from build123d import *

# Parameters (mm, degrees)
F1_DEPTH = 3.175
F2_R     = 38.608
F2_R_2   = 36.322
F2_R_3   = 11.1633
F3_DEPTH = 1.524
F4_R     = 0.5334
F5_DEPTH = 3.176


with BuildPart() as f1:
    # F0 (on Top) → F1 (new body)
    with BuildSketch(Plane.XY):
        Polygon((18.411793, 44.45), (-18.411793, 44.45), (-44.45, 18.411793), (-44.45, 0), (44.45, 0), (44.45, 18.411793), align=None)
        Polygon((44.45, 0), (-44.45, 0), (-44.45, -18.411793), (-18.411793, -44.45), (18.411793, -44.45), (44.45, -18.411793), align=None)
    extrude(amount=F1_DEPTH)

    # F2 (on face) → F3 (cut)
    with BuildSketch(Plane.XY.offset(3.175)):
        Circle(F2_R)
        Circle(F2_R_2, mode=Mode.SUBTRACT)
        Circle(F2_R_3)
    extrude(amount=-F3_DEPTH, mode=Mode.SUBTRACT)

    # F4 (on Top) → F5 (cut, through all)
    with BuildSketch(Plane.XY):
        with Locations((0, -13.6967)):
            Circle(F4_R)
        with Locations((0, -15.6967)):
            Circle(F4_R)
        with Locations((0, -17.6967)):
            Circle(F4_R)
        with Locations((0, -19.6967)):
            Circle(F4_R)
        with Locations((0, -21.6967)):
            Circle(F4_R)
        with Locations((0, -23.6967)):
            Circle(F4_R)
        with Locations((-8.977923, -8.977923)):
            Circle(F4_R)
        with Locations((-10.392136, -10.392136)):
            Circle(F4_R)
        with Locations((-11.80635, -11.80635)):
            Circle(F4_R)
        with Locations((-13.220563, -13.220563)):
            Circle(F4_R)
        with Locations((-14.634777, -14.634777)):
            Circle(F4_R)
        with Locations((-16.04899, -16.04899)):
            Circle(F4_R)
        with Locations((-21.6967, 0)):
            Circle(F4_R)
        with Locations((-23.6967, 0)):
            Circle(F4_R)
        with Locations((-13.6967, 0)):
            Circle(F4_R)
        with Locations((-17.6967, 0)):
            Circle(F4_R)
        with Locations((-15.6967, 0)):
            Circle(F4_R)
        with Locations((-19.6967, 0)):
            Circle(F4_R)
        with Locations((-16.04899, 16.04899)):
            Circle(F4_R)
        with Locations((-14.634777, 14.634777)):
            Circle(F4_R)
        with Locations((-8.977923, 8.977923)):
            Circle(F4_R)
        with Locations((-10.392136, 10.392136)):
            Circle(F4_R)
        with Locations((-13.220563, 13.220563)):
            Circle(F4_R)
        with Locations((-11.80635, 11.80635)):
            Circle(F4_R)
        with Locations((0, 21.6967)):
            Circle(F4_R)
        with Locations((0, 23.6967)):
            Circle(F4_R)
        with Locations((0, 13.6967)):
            Circle(F4_R)
        with Locations((0, 17.6967)):
            Circle(F4_R)
        with Locations((0, 15.6967)):
            Circle(F4_R)
        with Locations((0, 19.6967)):
            Circle(F4_R)
        with Locations((16.04899, 16.04899)):
            Circle(F4_R)
        with Locations((14.634777, 14.634777)):
            Circle(F4_R)
        with Locations((8.977923, 8.977923)):
            Circle(F4_R)
        with Locations((10.392136, 10.392136)):
            Circle(F4_R)
        with Locations((13.220563, 13.220563)):
            Circle(F4_R)
        with Locations((11.80635, 11.80635)):
            Circle(F4_R)
        with Locations((21.6967, 0)):
            Circle(F4_R)
        with Locations((23.6967, 0)):
            Circle(F4_R)
        with Locations((13.6967, 0)):
            Circle(F4_R)
        with Locations((17.6967, 0)):
            Circle(F4_R)
        with Locations((15.6967, 0)):
            Circle(F4_R)
        with Locations((19.6967, 0)):
            Circle(F4_R)
        with Locations((16.04899, -16.04899)):
            Circle(F4_R)
        with Locations((14.634777, -14.634777)):
            Circle(F4_R)
        with Locations((8.977923, -8.977923)):
            Circle(F4_R)
        with Locations((10.392136, -10.392136)):
            Circle(F4_R)
        with Locations((13.220563, -13.220563)):
            Circle(F4_R)
        with Locations((11.80635, -11.80635)):
            Circle(F4_R)
    extrude(amount=F5_DEPTH, mode=Mode.SUBTRACT)


solid = f1.part
Here's how the part is built. I have some questions about the finished solid (model axes, mm). A direction names the side the tool comes from. Coordinates: 2 decimals unless noted, no trailing zeros. Order: outer loops, then holes, each group sorted by start corner. A loop starts at its lowest first (then second) coordinate and runs counter-clockwise, first axis right, second up.
Item 1: If we section it at D-D on z = 0.5: State how many separate pieces and enclosed holes the cut face has, plus the area to 3 significant figures.
Result sheet:
separate pieces: 1
enclosed holes: 48
area: 6,500 mm2
Item 2: I need wall thicknesses on line 1 (X direction, y = -10.5, z = 1.5); line 2 (Y direction, x = -7, z = 2); line 3 (Y direction, x = 5.5, z = 2.5). Which ranges of each line are inside material? Lowest first, please.
Result sheet:
line 1: x = -44.45 to -10.91, -9.87 to 9.87, 10.91 to 44.45
line 2: y = -44.45 to -37.97, -35.64 to -8.7, 8.7 to 35.64, 37.97 to 44.45
line 3: y = -44.45 to -38.21, -35.9 to -9.71, 9.71 to 35.9, 38.21 to 44.45
Item 3: If we section it at A-A on y = -2: List the corners of the cut face in (x, z) for me (3 decimals), plus the area to 3 significant figures.
Result sheet:
outline: (-44.45, 0) - (44.45, 0) - (44.45, 3.175) - (38.556, 3.175) - (38.556, 1.651) - (36.267, 1.651) - (36.267, 3.175) - (10.983, 3.175) - (10.983, 1.651) - (-10.983, 1.651) - (-10.983, 3.175) - (-36.267, 3.175) - (-36.267, 1.651) - (-38.556, 1.651) - (-38.556, 3.175) - (-44.45, 3.175) - close
area: 242 mm2
Item 4: For faces 1 (the face through (-1, 1, 0)), 2 (the face through (0, 0, 1.651)), which set-ups out of +Z, -Z, +X, -X, +Y, -Y let a thin tool reach every point of the face, with its end or its side?
Result sheet:
face 1: -Z, +X, -X, +Y, -Y
face 2: +Z
Item 5: For P1, Ø0.6, axis at x = -8.98, y = 8.98, coming from the -Z side; P2, Ø1.5, axis at x = 30.5, z = 1, coming from the -Y side, each with a flat end and sliding along its axis, tell me the tip position at first contact or that it passes through.
Result sheet:
P1: passes through
P2: stops at y = -33.11
Item 6: If we mould it in two halves opening along X, with no side actions, what happens to faces 3 (the face through (-31.61, -31.25, 1.57)), 4 (the face through (19.526, 30.627, 2.424)), 5 (the face through (44.45, 0, 2))? For each: +X half, -X half, draft (parallel to the pull), parting line (faces both ways), or undercut.
Result sheet:
face 3: -X half
face 4: undercut
face 5: +X half
Item 7: If we section it at B-B on x = -26.5: List the corners of the cut face in (y, z) for me (3 decimals).
Result sheet:
outline: (-36.362, 0) - (36.362, 0) - (36.362, 3.175) - (28.077, 3.175) - (28.077, 1.651) - (24.84, 1.651) - (24.84, 3.175) - (-24.84, 3.175) - (-24.84, 1.651) - (-28.077, 1.651) - (-28.077, 3.175) - (-36.362, 3.175) - close
